```python
from build123d import *

# Parameters (mm, degrees)
BOSS_EXTRUDE1_DEPTH = 50
SKETCH2_R           = 60
CUT_EXTRUDE1_DEPTH  = 13
SKETCH3_R           = 10
CUT_EXTRUDE2_DEPTH  = 50
SKETCH4_R           = 2
BOSS_EXTRUDE2_DEPTH = 13
CUT_EXTRUDE3_DEPTH  = 30
SKETCH6_R           = 6
BOSS_EXTRUDE4_DEPTH = 3
SKETCH7_R           = 30
CUT_EXTRUDE4_DEPTH  = 40


with BuildPart() as part:
    # Sketch1 → Boss-Extrude1 (new body)
    with BuildSketch(Plane(origin=(0, 0, 0), x_dir=(1, 0, 0), z_dir=(0, 1, 0))):
        with BuildLine():
            Line((-57.148676171, 55.458248473), (62.851323829, 55.458248473))
            ThreePointArc((62.851323829, 55.458248473), (69.922391641, 52.529316284), (72.851323829, 45.458248473))
            Line((72.851323829, 45.458248473), (72.851323829, -74.541751527))
            ThreePointArc((72.851323829, -74.541751527), (69.922391641, -81.612819339), (62.851323829, -84.541751527))
            Line((62.851323829, -84.541751527), (-57.148676171, -84.541751527))
            ThreePointArc((-57.148676171, -84.541751527), (-64.219743983, -81.612819339), (-67.148676171, -74.541751527))
            Line((-67.148676171, -74.541751527), (-67.148676171, 45.458248473))
            ThreePointArc((-67.148676171, 45.458248473), (-64.219743983, 52.529316284), (-57.148676171, 55.458248473))
        make_face()
    extrude(amount=BOSS_EXTRUDE1_DEPTH)

    # Sketch2 → Cut-Extrude1 (cut)
    with BuildSketch(Plane(origin=(0, 50, 0), x_dir=(1, 0, 0), z_dir=(0, 1, 0))):
        with Locations(Location((2.851323829, -14.541751527, 0), (0, 0, 270))):
            Circle(SKETCH2_R)
    extrude(amount=-CUT_EXTRUDE1_DEPTH, mode=Mode.SUBTRACT)

    # Sketch3 → Cut-Extrude2 (cut)
    with BuildSketch(Plane(origin=(0, 37, 0), x_dir=(1, 0, 0), z_dir=(0, 1, 0))):
        with Locations(Location((2.851323829, -14.541751527, 0), (0, 0, 270))):
            Circle(SKETCH3_R)
    extrude(amount=-CUT_EXTRUDE2_DEPTH, mode=Mode.SUBTRACT)

    # Sketch4 → Boss-Extrude2 (add)
    with BuildSketch(Plane(origin=(0, 37, 0), x_dir=(1, 0, 0), z_dir=(0, 1, 0))):
        with Locations(Location((2.851323829, 33.458248473, 0), (0, 0, 90))):
            Circle(SKETCH4_R)
        with Locations(Location((36.792449326, 19.399373969, 0), (0, 0, 90))):
            Circle(SKETCH4_R)
        with Locations(Location((50.851323829, -14.541751527, 0), (0, 0, 90))):
            Circle(SKETCH4_R)
        with Locations(Location((36.792449326, -48.482877024, 0), (0, 0, 90))):
            Circle(SKETCH4_R)
        with Locations(Location((2.851323829, -62.541751527, 0), (0, 0, 90))):
            Circle(SKETCH4_R)
        with Locations(Location((-31.089801668, -48.482877024, 0), (0, 0, 90))):
            Circle(SKETCH4_R)
        with Locations(Location((-45.148676171, -14.541751527, 0), (0, 0, 90))):
            Circle(SKETCH4_R)
        with Locations(Location((-31.089801668, 19.399373969, 0), (0, 0, 90))):
            Circle(SKETCH4_R)
    extrude(amount=BOSS_EXTRUDE2_DEPTH)

    # Sketch5 → Cut-Extrude3 (cut)
    with BuildSketch(Plane.XZ):
        with BuildLine():
            Line((-37.148676171, 64.541751527), (42.851323829, 64.541751527))
            ThreePointArc((42.851323829, 64.541751527), (49.922391641, 61.612819339), (52.851323829, 54.541751527))
            Line((52.851323829, 54.541751527), (52.851323829, -25.458248473))
            ThreePointArc((52.851323829, -25.458248473), (49.922391641, -32.529316284), (42.851323829, -35.458248473))
            Line((42.851323829, -35.458248473), (-37.148676171, -35.458248473))
            ThreePointArc((-37.148676171, -35.458248473), (-44.219743983, -32.529316284), (-47.148676171, -25.458248473))
            Line((-47.148676171, -25.458248473), (-47.148676171, 54.541751527))
            ThreePointArc((-47.148676171, 54.541751527), (-44.219743983, 61.612819339), (-37.148676171, 64.541751527))
        make_face()
    extrude(amount=-CUT_EXTRUDE3_DEPTH, mode=Mode.SUBTRACT)

    # Sketch6 → Boss-Extrude4 (add)
    with BuildSketch(Plane.XZ):
        with Locations(Location((-57.148676171, 74.541751527, 0), (0, 0, 90))):
            Circle(SKETCH6_R)
        with Locations(Location((62.851323829, 74.541751527, 0), (0, 0, 90))):
            Circle(SKETCH6_R)
        with Locations(Location((62.851323829, -45.458248473, 0), (0, 0, 90))):
            Circle(SKETCH6_R)
        with Locations(Location((-57.148676171, -45.458248473, 0), (0, 0, 90))):
            Circle(SKETCH6_R)
    extrude(amount=BOSS_EXTRUDE4_DEPTH)

    # Sketch7 → Cut-Extrude4 (cut)
    with BuildSketch(Plane(origin=(0, 37, 0), x_dir=(1, 0, 0), z_dir=(0, 1, 0))):
        with Locations(Location((2.851323829, -14.541751527, 0), (0, 0, 270))):
            Circle(SKETCH7_R)
    extrude(amount=-CUT_EXTRUDE4_DEPTH, mode=Mode.SUBTRACT)


solid = part.part
```
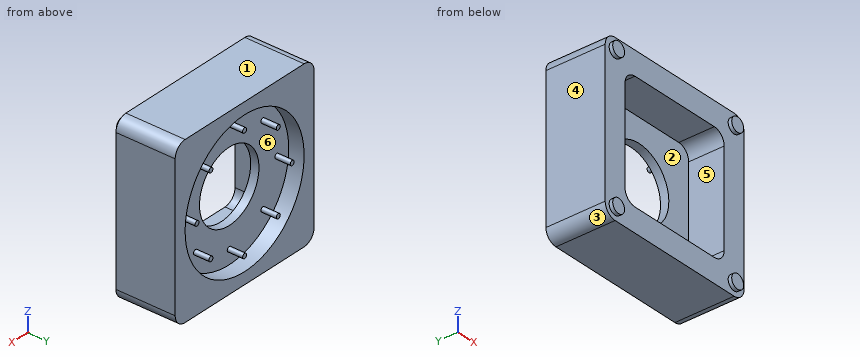
Could you check a few things on this model? Use its own coordinates, in mm. Face numbers are marked on the shaded views. A direction names the side the tool comes from. Coordinates: 2 decimals unless noted, no trailing zeros. Loops run counter-clockwise (first coordinate to the right, second up) from the corner with the lowest first, then second, coordinate; pieces in that order, holes last.
1) Imagine slicing it at D-D (z = -13). List the corners of the cut face in (x, y) for me, and give its area (3 significant figures).
Reported:
outline: (-67.15, 0) - (-47.15, 0) - (-47.15, 30) - (-9.04, 30) - (-9.04, 37) - (-50.45, 37) - (-50.45, 50) - (-67.15, 50) - close; (14.74, 30) - (52.85, 30) - (52.85, 0) - (72.85, 0) - (72.85, 50) - (56.16, 50) - (56.16, 37) - (14.74, 37) - close
area: 2,450 mm2
2) Imagine slicing it at A-A (y = 11). List the corners of the cut face in (x, z) for me.
Reported:
outline: (-67.15, -45.46) arc R10 ccw to (-57.15, -55.46) - (62.85, -55.46) arc R10 ccw to (72.85, -45.46) - (72.85, 74.54) arc R10 ccw to (62.85, 84.54) - (-57.15, 84.54) arc R10 ccw to (-67.15, 74.54) - close; hole (-47.15, -25.46) arc R10 ccw to (-37.15, -35.46) - (42.85, -35.46) arc R10 ccw to (52.85, -25.46) - (52.85, 54.54) arc R10 ccw to (42.85, 64.54) - (-37.15, 64.54) arc R10 ccw to (-47.15, 54.54) - close
3) Imagine slicing it at C-C (x = 21). List the corners of the cut face in (y, z) for me, and give its area (3 significant figures).
Reported:
outline: (0, -55.46) - (50, -55.46) - (50, -42.65) - (37, -42.65) - (37, -9.35) - (30, -9.35) - (30, -35.46) - (0, -35.46) - close; (0, 64.54) - (30, 64.54) - (30, 38.43) - (37, 38.43) - (37, 71.73) - (50, 71.73) - (50, 84.54) - (0, 84.54) - close
area: 2,180 mm2
4) Which directions (+Z, -Z, +X, -X, +Y, -Y) give clear straight access to the entire face, cutting with the end or side of a thin tool? Please do the marked faces 4, 5 and 6.
Reported:
face 4: +Z, -Z, -X, +Y, -Y
face 5: -Y
face 6: +Y
5) Imagine slicing it at B-B (y = 41). State how many separate pieces and enclosed holes the cut face has, and give its area (3 significant figures).
Reported:
separate pieces: 9
enclosed holes: 1
area: 8,300 mm2
6) Will these pins go through, and if not, where does the flat tip stop? pin 1 Ø4 at (x, z) = (-28, -22.5) entering from +Y; pin 2 Ø12 at (x, z) = (-24.5, 54) entering from -Y.
Reported:
pin 1: stops at y = 37
pin 2: stops at y = 30
7) Please list where these lines run through material, in increasing order: line 1 along X through (y, z) = (21, 14.5); line 2 along Z through (x, y) = (24, 14); line 3 along Y through (x, z) = (54, 74.5).
Reported:
line 1: x = -67.15 to -47.15, 52.85 to 72.85
line 2: z = -55.46 to -35.46, 64.54 to 84.54
line 3: y = 0 to 50
8) Thinking about a two-plate mould opening in X: for the marked faces 1, 2 and 3, which applies, released by +X, released by -X, zero draft, split by the parting line, or undercut?
Reported:
face 1: zero draft
face 2: undercut
face 3: released by -X
